Autodesk Inventor part; units mm, degrees
ref_plane "YZ Plane" through (0, 0, 0) normal (1, 0, 0) x (0, 1, 0)
ref_plane "XZ Plane" through (0, 0, 0) normal (0, 1, 0) x (-1, 0, 0)
ref_plane "XY Plane" through (0, 0, 0) normal (0, 0, 1) x (1, 0, 0)
sketch "Sketch1" plane through (0, 0, 0) normal (0, 0, 1) x (1, 0, 0)
  line L0 (-12.7, -25.4) -> (12.7, -25.4)
  line L1 (12.7, -25.4) -> (12.7, 25.4)
  line L2 (12.7, 25.4) -> (-12.7, 25.4)
  line L3 (-12.7, 25.4) -> (-12.7, -25.4)
  line L4 (-12.7, -25.4) -> (12.7, 25.4) construction
  line L5 (12.7, -25.4) -> (-12.7, 25.4) construction
  line L6 (-11.1125, 23.8125) -> (11.1125, 23.8125)
  line L7 (11.1125, 23.8125) -> (11.1125, -23.8125)
  line L8 (11.1125, -23.8125) -> (-11.1125, -23.8125)
  line L9 (-11.1125, -23.8125) -> (-11.1125, 23.8125)
  point P0 (0, 0)
  dimension "width" = 25.4
  dimension "height" = 50.8
  dimension "thickness" = 1.5875
extrude "Extrusion1" add sketch "Sketch1" along normal mid plane 304.8
sketch "Sketch2" plane through (-12.7, -25.4, 152.4) normal (-1, 0, 0) x (0, 0, 1)
  line L0 (-292.1, 44.45) -> (-292.1, 6.35) construction
  line L1 (-304.8, 0) -> (-304.8, 50.8) construction
  line L2 (0, 50.8) -> (0, 0) construction
  point P0 (-152.4, 25.4)
  point P1 (-12.7, 6.35)
  point P2 (-12.7, 44.45)
  point P3 (-292.1, 25.4)
  dimension "d5" = 12.7
  dimension "d6" = 12.7
  dimension "d7" = 38.1
hole "Hole1" at (-12.7, 19.05, -139.7) at (-12.7, -19.05, -139.7) at (-12.7, -19.05, 139.7) at (-12.7, 19.05, 139.7) direction (1, 0, 0) diameter 5.1054 end through all
properties part number "CL7-015" material "Aluminum 6061"
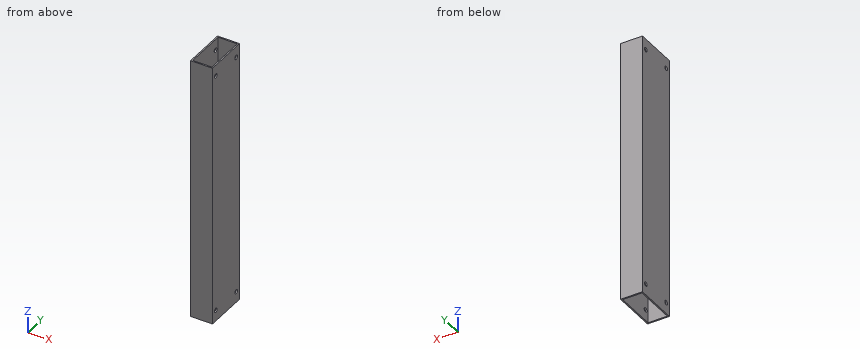
Can you work these out from the model? Positions are in its coordinate system, mm. Coordinates: 2 decimals unless noted, no trailing zeros. Write each loop counter-clockwise with the first axis right and the second up, starting at its lowest first coordinate (ties: lowest second). Pieces come first, ordered by that corner, then holes.
Q1. Imagine slicing it at A-A, the plane z = 139.7. List the corners of the cut face in (x, y) for me.
Results found:
outline: (-12.7, -25.4) - (12.7, -25.4) - (12.7, -21.6) - (11.11, -21.6) - (11.11, -23.81) - (-11.11, -23.81) - (-11.11, -21.6) - (-12.7, -21.6) - close; (-12.7, -16.5) - (-11.11, -16.5) - (-11.11, 16.5) - (-12.7, 16.5) - close; (-12.7, 21.6) - (-11.11, 21.6) - (-11.11, 23.81) - (11.11, 23.81) - (11.11, 21.6) - (12.7, 21.6) - (12.7, 25.4) - (-12.7, 25.4) - close; (11.11, -16.5) - (12.7, -16.5) - (12.7, 16.5) - (11.11, 16.5) - close
Q2. Imagine slicing it at B-B, the plane y = 19.05. List the corners of the cut face in (x, z) for me.
Results found:
outline: (-12.7, -152.4) - (-11.11, -152.4) - (-11.11, -142.25) - (-12.7, -142.25) - close; (-12.7, -137.15) - (-11.11, -137.15) - (-11.11, 137.15) - (-12.7, 137.15) - close; (-12.7, 142.25) - (-11.11, 142.25) - (-11.11, 152.4) - (-12.7, 152.4) - close; (11.11, -152.4) - (12.7, -152.4) - (12.7, -142.25) - (11.11, -142.25) - close; (11.11, -137.15) - (12.7, -137.15) - (12.7, 137.15) - (11.11, 137.15) - close; (11.11, 142.25) - (12.7, 142.25) - (12.7, 152.4) - (11.11, 152.4) - close
Q3. Imagine slicing it at C-C, the plane x = -7.5. List the corners of the cut face in (y, z) for me, plus the area to 3 significant figures.
Results found:
outline: (-25.4, -152.4) - (-23.81, -152.4) - (-23.81, 152.4) - (-25.4, 152.4) - close; (23.81, -152.4) - (25.4, -152.4) - (25.4, 152.4) - (23.81, 152.4) - close
area: 968 mm2
Q4. Imagine slicing it at D-D, the plane z = 102. List the corners of the cut face in (x, y) for me.
Results found:
outline: (-12.7, -25.4) - (12.7, -25.4) - (12.7, 25.4) - (-12.7, 25.4) - close; hole (-11.11, -23.81) - (11.11, -23.81) - (11.11, 23.81) - (-11.11, 23.81) - close
Q5. Please list where these lines run through material, in increasing order: L1, parallel to Y at x = -11.5, z = -139.7; L2, parallel to Z at x = -11.8, y = 19.05; L3, parallel to Y at x = -3.5, z = 46.5.
Results found:
L1: y = -25.4 to -21.6, -16.5 to 16.5, 21.6 to 25.4
L2: z = -152.4 to -142.25, -137.15 to 137.15, 142.25 to 152.4
L3: y = -25.4 to -23.81, 23.81 to 25.4
Q6. For P1, Ø3, axis at y = -19.05, z = -139.7, coming from the +X side, with a flat end and sliding along its axis, tell me the tip position at first contact or that it passes through.
Results found:
P1: passes through
